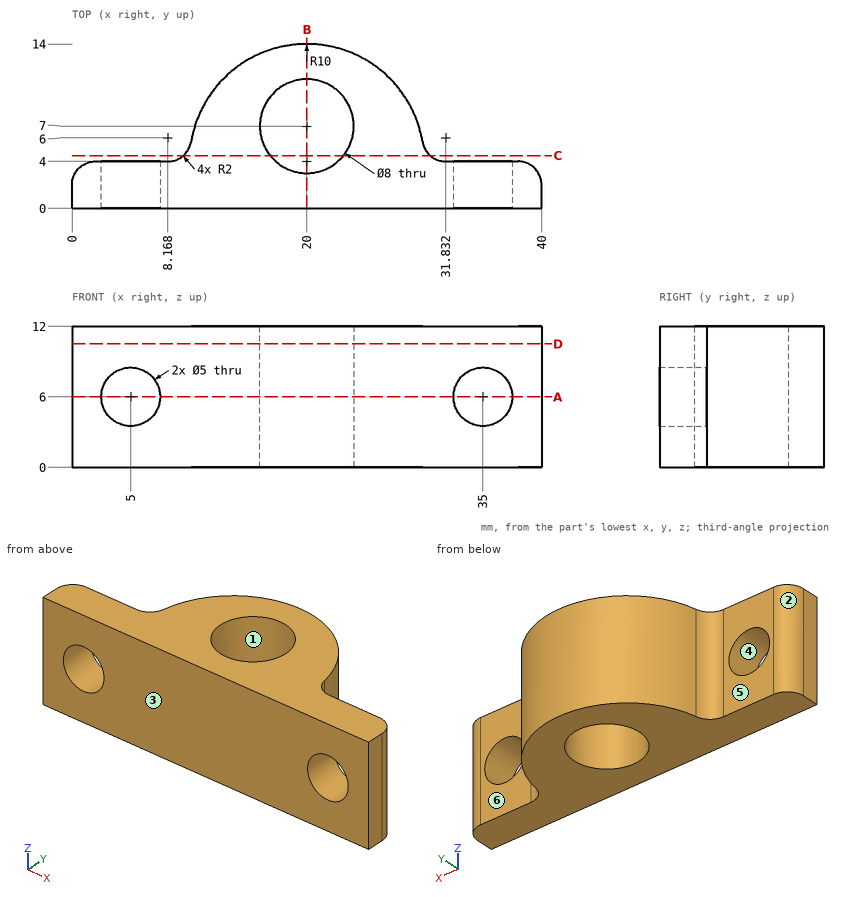
Geometry: see drawing. Coordinates: mm, zero at the bounding-box minimum. A direction names the side the tool comes from. Coordinates: 2 decimals unless noted, no trailing zeros. Order: outer loops, then holes, each group sorted by start corner. A loop starts at its lowest first (then second) coordinate and runs counter-clockwise, first axis right, second up. Notation, with made-up numbers: (72, -19.5) - (100, -19.5) arc R16 ccw to (100, 4.5) - close; hole circle Ø11 at (41, 12.25). An arc over 180 degrees is marked (long way). Return JSON: item names as keys, results as strings.
Q1. First-contact query: pin 1 (2 mm diameter, centred on x = 14, z = 7, fed in from +Y); pin 2 (1.5 mm diameter, centred on y = 10.5, z = 4.5, fed in from +X); pin 3 (5 mm diameter, centred on x = 35.5, z = 3.5, fed in from +Y). Flat tips, straight axial feed; report the tip coordinate or a pass-through.
The answers:
{"pin 1": "stops at y = 12.66", "pin 2": "stops at x = 28.18", "pin 3": "stops at y = 4"}
Q2. Cut plane C-C (y = 4.5). Return loops of the section in (x, z), then the cut area to 3 significant figures.
The answers:
{"outline": "(9.49, 0) - (16.88, 0) - (16.88, 12) - (9.49, 12) - close; (23.12, 0) - (30.51, 0) - (30.51, 12) - (23.12, 12) - close", "area": "177 mm2"}
Q3. Draft query along Y for the marked faces 1, 2 and 3. Return one class per face: +Y half, -Y half, draft (parallel to the pull), parting line (faces both ways), or undercut.
The answers:
{"face 1": "undercut", "face 2": "+Y half", "face 3": "-Y half"}
Q4. Cut plane D-D (z = 10.5). Return loops of the section in (x, y).
The answers:
{"outline": "(0, 0) - (40, 0) - (40, 2) arc R2 ccw to (38, 4) - (31.83, 4) arc R2 cw to (29.86, 5.67) arc R10 ccw to (10.14, 5.67) arc R2 cw to (8.17, 4) - (2, 4) arc R2 ccw to (0, 2) - close; hole circle Ø8 at (20, 7)"}
Q5. Cut plane A-A (z = 6). Return loops of the section in (x, y), then the cut area to 3 significant figures.
The answers:
{"outline": "(0, 0) - (2.5, 0) - (2.5, 4) - (2, 4) arc R2 ccw to (0, 2) - close; (7.5, 0) - (32.5, 0) - (32.5, 4) - (31.83, 4) arc R2 cw to (29.86, 5.67) arc R10 ccw to (10.14, 5.67) arc R2 cw to (8.17, 4) - (7.5, 4) - close; (37.5, 0) - (40, 0) - (40, 2) arc R2 ccw to (38, 4) - (37.5, 4) - close; hole circle Ø8 at (20, 7)", "area": "226 mm2"}
Q6. Ray query, probe 1 along Z at (x, y) = (5, 1.85); probe 2 along X at (y, z) = (2.6, 6); probe 3 along Y at (x, z) = (35, 1.75). Return the intervals inside material, ascending.
The answers:
{"probe 1": "z = 0 to 3.5, 8.5 to 12", "probe 2": "x = 0.09 to 2.5, 7.5 to 32.5, 37.5 to 39.91", "probe 3": "y = 0 to 4"}
Q7. Cut plane B-B (x = 20). Return loops of the section in (y, z).
The answers:
{"outline": "(0, 0) - (3, 0) - (3, 12) - (0, 12) - close; (11, 0) - (14, 0) - (14, 12) - (11, 12) - close"}
Q8. Access query for the marked faces 4, 5 and 6. Directions: +Z, -Z, +X, -X, +Y, -Y. A direction counts if a zero-diameter tool reaches every point of the face in a straight line with its end or side. Return the directions, or none.
The answers:
{"face 4": "+Y, -Y", "face 5": "+Z, -Z, -X, +Y", "face 6": "+Z, -Z, +X, +Y"}
